from build123d import *

# Parameters (mm, degrees)
EXTRUDE_THIN1_DEPTH       = 350
FILLET1_R                 = 1.2
CUT_EXTRUDE1_DEPTH        = 26
LPATTERN1_COUNT           = 14
LPATTERN1_PITCH           = 28
CIRPATTERN1_COUNT         = 2
CIRPATTERN1_ANGLE         = 270
CIRPATTERN1_COPY_1_DEPTH  = 26
CIRPATTERN1_COPY_2_DEPTH  = 26
CIRPATTERN1_COPY_3_DEPTH  = 26
CIRPATTERN1_COPY_4_DEPTH  = 26
CIRPATTERN1_COPY_5_DEPTH  = 26
CIRPATTERN1_COPY_6_DEPTH  = 26
CIRPATTERN1_COPY_7_DEPTH  = 26
CIRPATTERN1_COPY_8_DEPTH  = 26
CIRPATTERN1_COPY_9_DEPTH  = 26
CIRPATTERN1_COPY_10_DEPTH = 26
CIRPATTERN1_COPY_11_DEPTH = 26
CIRPATTERN1_COPY_12_DEPTH = 26
CIRPATTERN1_COPY_13_DEPTH = 26
SKETCH5_W                 = 1.2
SKETCH5_H                 = 7
SKETCH5_H_2               = 10.2
SKETCH5_W_2               = 9
SKETCH5_H_3               = 1.2
CUT_EXTRUDE3_DEPTH        = 16


with BuildPart() as part:
    # Sketch1 → Extrude-Thin1 (new body)
    with BuildSketch(Plane(origin=(0, 0, 0), x_dir=(1, 0, 0), z_dir=(0, 1, 0))):
        Polygon((25, 0), (0, 0), (0, 25), (1.2, 25), (1.2, 1.2), (25, 1.2), align=None)
    extrude(amount=EXTRUDE_THIN1_DEPTH)

    # Fillet1
    fillet1_edges = [part.edges().sort_by_distance(p)[0] for p in [
        (0, 175, 0),
        (1.2, 175, -1.2),
    ]]
    fillet(fillet1_edges, radius=FILLET1_R)

    # Sketch2 → Cut-Extrude1 (cut, through all)
    with BuildSketch(Plane.XY):
        with BuildLine():
            Line((9, 9.5), (9, 16.5))
            ThreePointArc((9, 16.5), (12.5, 20), (16, 16.5))
            Line((16, 16.5), (16, 9.5))
            ThreePointArc((16, 9.5), (12.5, 6), (9, 9.5))
        make_face()
    cut_extrude1 = extrude(amount=-CUT_EXTRUDE1_DEPTH, mode=Mode.SUBTRACT)

    # LPattern1: Cut-Extrude1 ×14
    with Locations(*[(0, i * LPATTERN1_PITCH, 0) for i in range(1, LPATTERN1_COUNT)]):
        add(cut_extrude1, mode=Mode.SUBTRACT)

    # CirPattern1: Cut-Extrude1 ×2 about axis
    cirpattern1_axis = Axis((1.2, 350, 0), (0, -1, 0))
    for i in range(1, CIRPATTERN1_COUNT):
        add(cut_extrude1.rotate(cirpattern1_axis, i * CIRPATTERN1_ANGLE / (CIRPATTERN1_COUNT - 1)), mode=Mode.SUBTRACT)

    # CirPattern1 copy 1 sketch → CirPattern1 copy 1 (cut, through all)
    with BuildSketch(Plane(origin=(1.2, 28, 1.2), x_dir=(0, 0, -1), z_dir=(1, 0, 0))):
        with BuildLine():
            Line((9, 9.5), (9, 16.5))
            ThreePointArc((9, 16.5), (12.5, 20), (16, 16.5))
            Line((16, 16.5), (16, 9.5))
            ThreePointArc((16, 9.5), (12.5, 6), (9, 9.5))
        make_face()
    extrude(amount=-CIRPATTERN1_COPY_1_DEPTH, mode=Mode.SUBTRACT)

    # CirPattern1 copy 2 sketch → CirPattern1 copy 2 (cut, through all)
    with BuildSketch(Plane(origin=(1.2, 56, 1.2), x_dir=(0, 0, -1), z_dir=(1, 0, 0))):
        with BuildLine():
            Line((9, 9.5), (9, 16.5))
            ThreePointArc((9, 16.5), (12.5, 20), (16, 16.5))
            Line((16, 16.5), (16, 9.5))
            ThreePointArc((16, 9.5), (12.5, 6), (9, 9.5))
        make_face()
    extrude(amount=-CIRPATTERN1_COPY_2_DEPTH, mode=Mode.SUBTRACT)

    # CirPattern1 copy 3 sketch → CirPattern1 copy 3 (cut, through all)
    with BuildSketch(Plane(origin=(1.2, 84, 1.2), x_dir=(0, 0, -1), z_dir=(1, 0, 0))):
        with BuildLine():
            Line((9, 9.5), (9, 16.5))
            ThreePointArc((9, 16.5), (12.5, 20), (16, 16.5))
            Line((16, 16.5), (16, 9.5))
            ThreePointArc((16, 9.5), (12.5, 6), (9, 9.5))
        make_face()
    extrude(amount=-CIRPATTERN1_COPY_3_DEPTH, mode=Mode.SUBTRACT)

    # CirPattern1 copy 4 sketch → CirPattern1 copy 4 (cut, through all)
    with BuildSketch(Plane(origin=(1.2, 112, 1.2), x_dir=(0, 0, -1), z_dir=(1, 0, 0))):
        with BuildLine():
            Line((9, 9.5), (9, 16.5))
            ThreePointArc((9, 16.5), (12.5, 20), (16, 16.5))
            Line((16, 16.5), (16, 9.5))
            ThreePointArc((16, 9.5), (12.5, 6), (9, 9.5))
        make_face()
    extrude(amount=-CIRPATTERN1_COPY_4_DEPTH, mode=Mode.SUBTRACT)

    # CirPattern1 copy 5 sketch → CirPattern1 copy 5 (cut, through all)
    with BuildSketch(Plane(origin=(1.2, 140, 1.2), x_dir=(0, 0, -1), z_dir=(1, 0, 0))):
        with BuildLine():
            Line((9, 9.5), (9, 16.5))
            ThreePointArc((9, 16.5), (12.5, 20), (16, 16.5))
            Line((16, 16.5), (16, 9.5))
            ThreePointArc((16, 9.5), (12.5, 6), (9, 9.5))
        make_face()
    extrude(amount=-CIRPATTERN1_COPY_5_DEPTH, mode=Mode.SUBTRACT)

    # CirPattern1 copy 6 sketch → CirPattern1 copy 6 (cut, through all)
    with BuildSketch(Plane(origin=(1.2, 168, 1.2), x_dir=(0, 0, -1), z_dir=(1, 0, 0))):
        with BuildLine():
            Line((9, 9.5), (9, 16.5))
            ThreePointArc((9, 16.5), (12.5, 20), (16, 16.5))
            Line((16, 16.5), (16, 9.5))
            ThreePointArc((16, 9.5), (12.5, 6), (9, 9.5))
        make_face()
    extrude(amount=-CIRPATTERN1_COPY_6_DEPTH, mode=Mode.SUBTRACT)

    # CirPattern1 copy 7 sketch → CirPattern1 copy 7 (cut, through all)
    with BuildSketch(Plane(origin=(1.2, 196, 1.2), x_dir=(0, 0, -1), z_dir=(1, 0, 0))):
        with BuildLine():
            Line((9, 9.5), (9, 16.5))
            ThreePointArc((9, 16.5), (12.5, 20), (16, 16.5))
            Line((16, 16.5), (16, 9.5))
            ThreePointArc((16, 9.5), (12.5, 6), (9, 9.5))
        make_face()
    extrude(amount=-CIRPATTERN1_COPY_7_DEPTH, mode=Mode.SUBTRACT)

    # CirPattern1 copy 8 sketch → CirPattern1 copy 8 (cut, through all)
    with BuildSketch(Plane(origin=(1.2, 224, 1.2), x_dir=(0, 0, -1), z_dir=(1, 0, 0))):
        with BuildLine():
            Line((9, 9.5), (9, 16.5))
            ThreePointArc((9, 16.5), (12.5, 20), (16, 16.5))
            Line((16, 16.5), (16, 9.5))
            ThreePointArc((16, 9.5), (12.5, 6), (9, 9.5))
        make_face()
    extrude(amount=-CIRPATTERN1_COPY_8_DEPTH, mode=Mode.SUBTRACT)

    # CirPattern1 copy 9 sketch → CirPattern1 copy 9 (cut, through all)
    with BuildSketch(Plane(origin=(1.2, 252, 1.2), x_dir=(0, 0, -1), z_dir=(1, 0, 0))):
        with BuildLine():
            Line((9, 9.5), (9, 16.5))
            ThreePointArc((9, 16.5), (12.5, 20), (16, 16.5))
            Line((16, 16.5), (16, 9.5))
            ThreePointArc((16, 9.5), (12.5, 6), (9, 9.5))
        make_face()
    extrude(amount=-CIRPATTERN1_COPY_9_DEPTH, mode=Mode.SUBTRACT)

    # CirPattern1 copy 10 sketch → CirPattern1 copy 10 (cut, through all)
    with BuildSketch(Plane(origin=(1.2, 280, 1.2), x_dir=(0, 0, -1), z_dir=(1, 0, 0))):
        with BuildLine():
            Line((9, 9.5), (9, 16.5))
            ThreePointArc((9, 16.5), (12.5, 20), (16, 16.5))
            Line((16, 16.5), (16, 9.5))
            ThreePointArc((16, 9.5), (12.5, 6), (9, 9.5))
        make_face()
    extrude(amount=-CIRPATTERN1_COPY_10_DEPTH, mode=Mode.SUBTRACT)

    # CirPattern1 copy 11 sketch → CirPattern1 copy 11 (cut, through all)
    with BuildSketch(Plane(origin=(1.2, 308, 1.2), x_dir=(0, 0, -1), z_dir=(1, 0, 0))):
        with BuildLine():
            Line((9, 9.5), (9, 16.5))
            ThreePointArc((9, 16.5), (12.5, 20), (16, 16.5))
            Line((16, 16.5), (16, 9.5))
            ThreePointArc((16, 9.5), (12.5, 6), (9, 9.5))
        make_face()
    extrude(amount=-CIRPATTERN1_COPY_11_DEPTH, mode=Mode.SUBTRACT)

    # CirPattern1 copy 12 sketch → CirPattern1 copy 12 (cut, through all)
    with BuildSketch(Plane(origin=(1.2, 336, 1.2), x_dir=(0, 0, -1), z_dir=(1, 0, 0))):
        with BuildLine():
            Line((9, 9.5), (9, 16.5))
            ThreePointArc((9, 16.5), (12.5, 20), (16, 16.5))
            Line((16, 16.5), (16, 9.5))
            ThreePointArc((16, 9.5), (12.5, 6), (9, 9.5))
        make_face()
    extrude(amount=-CIRPATTERN1_COPY_12_DEPTH, mode=Mode.SUBTRACT)

    # CirPattern1 copy 13 sketch → CirPattern1 copy 13 (cut, through all)
    with BuildSketch(Plane(origin=(1.2, 364, 1.2), x_dir=(0, 0, -1), z_dir=(1, 0, 0))):
        with BuildLine():
            Line((9, 9.5), (9, 16.5))
            ThreePointArc((9, 16.5), (12.5, 20), (16, 16.5))
            Line((16, 16.5), (16, 9.5))
            ThreePointArc((16, 9.5), (12.5, 6), (9, 9.5))
        make_face()
    extrude(amount=-CIRPATTERN1_COPY_13_DEPTH, mode=Mode.SUBTRACT)

    # Sketch5 → Cut-Extrude3 (cut)
    with BuildSketch(Plane(origin=(0, 350, 0), x_dir=(1, 0, 0), z_dir=(0, 1, 0))):
        with Locations((0.6, 11.3)):
            Rectangle(SKETCH5_W, SKETCH5_H)
        with Locations((0.6, 19.9)):
            Rectangle(SKETCH5_W, SKETCH5_H_2)
        with BuildLine():
            Line((1.2, 7.8), (0, 7.8))
            Line((0, 7.8), (0, 1.2))
            ThreePointArc((0, 1.2), (0.351471863, 0.351471863), (1.2, 0))
            Line((1.2, 0), (9, 0))
            Line((9, 0), (9, 1.2))
            Line((9, 1.2), (2.4, 1.2))
            ThreePointArc((2.4, 1.2), (1.551471863, 1.551471863), (1.2, 2.4))
            Line((1.2, 2.4), (1.2, 7.8))
        make_face()
        Polygon((9, 1.2), (9, 0), (16, 0), (16, 1.2), (10.440408388, 1.2), align=None)
        with Locations((20.5, 0.6)):
            Rectangle(SKETCH5_W_2, SKETCH5_H_3)
    extrude(amount=-CUT_EXTRUDE3_DEPTH, mode=Mode.SUBTRACT)


solid = part.part
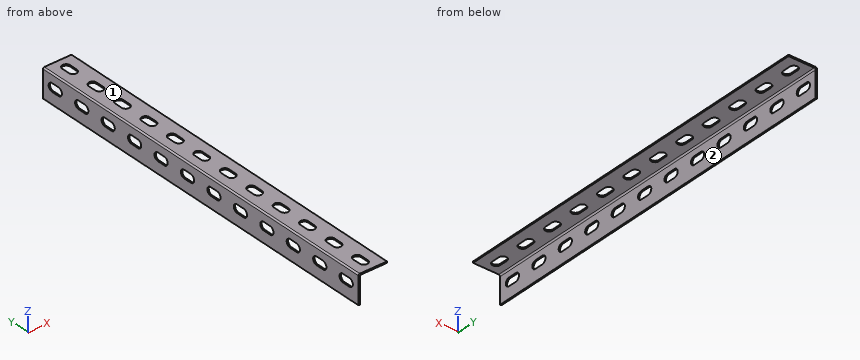
Geometry: final body of the model. Coordinates: model frame, mm. Face numbers are marked on the shaded views. A direction names the side the tool comes from. Give positions to 0.01 mm unless a question says otherwise; leave off trailing zeros. Order: outer loops, then holes, each group sorted by start corner. A loop starts at its lowest first (then second) coordinate and runs counter-clockwise, first axis right, second up. Notation, with made-up numbers: (1.25, 68) -> (55.25, 68) arc R20 cw to (55.25, 85) -> close; hole circle Ø8 at (-10, 60.25). An arc over 180 degrees is marked (long way). Answer as a JSON object with one key per item and string values.
Q1. Section A-A (y = 197.5). Output: boundary loops of the cut face in (x, z), plus the area to 3 significant figures.
Entries:
{"outline": "(0, -25) -> (1.2, -25) -> (1.2, -2.4) arc R1.2 cw to (2.4, -1.2) -> (25, -1.2) -> (25, 0) -> (1.2, 0) arc R1.2 ccw to (0, -1.2) -> close", "area": "58.6 mm^2"}
Q2. Access query for the marked faces 1 and 2. Directions: +Z, -Z, +X, -X, +Y, -Y. A direction counts if a zero-diameter tool reaches every point of the face in a straight line with its end or side. Return the directions, or none.
Entries:
{"face 1": "+Z, +X, -X, +Y, -Y", "face 2": "-Z, +X, +Y, -Y"}
Q3. Material intervals for probe 1 along X at (y, z) = (182.5, -7); probe 2 along Z at (x, y) = (3, 318); probe 3 along X at (y, z) = (207.5, -1.75), sorted ascending.
Entries:
{"probe 1": "x = 0 to 1.2", "probe 2": "z = -1.2 to 0", "probe 3": "x = 0 to 1.39"}
Q4. Section B-B (x = 13). State how many separate pieces and enclosed holes the cut face has, plus the area to 3 significant figures.
Entries:
{"separate pieces": "13", "enclosed holes": "0", "area": "200 mm^2"}
Q5. First-contact query: pin 1 (1 mm diameter, centred on y = 42, z = -0.5, fed in from -X). Flat tip, straight axial feed; report the tip coordinate or a pass-through.
Entries:
{"pin 1": "stops at x = 0.02"}
